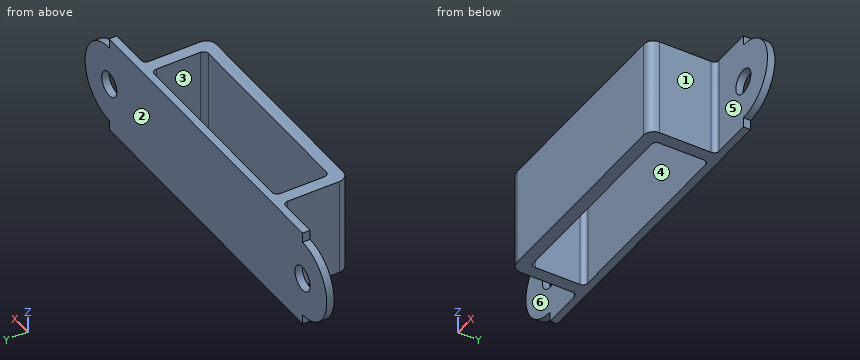
```python
from build123d import *

# Parameters (mm, degrees)
F0_W     = 46
F0_H     = 10
F1_DEPTH = 1.5
F2_DEPTH = 15
F3_W     = 41
F3_H     = 11
F4_DEPTH = 12.5
F5_D     = 5
F6_R     = 1
F7_R     = 2


with BuildPart() as f1:
    # F0 (on Front) → F1 (new body)
    with BuildSketch(Plane.XZ):
        with Locations((0, -5)):
            Rectangle(F0_W, F0_H)
        with Locations((0, 5)):
            Rectangle(F0_W, F0_H)
        Polygon((32, 10), (23, 10), (23, 0), (23, -10), (32, -10), (32, -8), (32, 8), align=None)
        with BuildLine():
            ThreePointArc((32, -8), (40, 0), (32, 8))
            Line((32, 8), (32, -8))
        make_face()
        Polygon((-23, 10), (-32, 10), (-32, 8), (-32, -8), (-32, -10), (-23, -10), (-23, 0), align=None)
        with BuildLine():
            Line((-32, -8), (-32, 8))
            ThreePointArc((-32, 8), (-40, 0), (-32, -8))
        make_face()
    extrude(amount=F1_DEPTH)

    # F0 (on Front) → F2 (join)
    with BuildSketch(Plane.XZ):
        with Locations((0, -5)):
            Rectangle(F0_W, F0_H)
        with Locations((0, 5)):
            Rectangle(F0_W, F0_H)
    extrude(amount=F2_DEPTH)

    # F3 (on Top) → F4 (cut, symmetric)
    with BuildSketch(Plane.XY):
        with Locations((0, -7)):
            Rectangle(F3_W, F3_H)
    extrude(amount=F4_DEPTH, both=True, mode=Mode.SUBTRACT)

    # F5 (through all)
    with Locations(Plane(origin=(0, 0, 0), x_dir=(1, 0, 0), z_dir=(0, 1, 0))):
        with Locations((-32, 0), (32, 0)):
            Hole(F5_D / 2)

    # F6
    f6_edges = [f1.edges().sort_by_distance(p)[0] for p in [
        (-23, -1.5, 0),
        (-20.5, -1.5, 0),
        (23, -1.5, 0),
        (20.5, -1.5, 0),
        (-20.5, -12.5, 0),
        (20.5, -12.5, 0),
    ]]
    fillet(f6_edges, radius=F6_R)

    # F7
    f7_edges = [f1.edges().sort_by_distance(p)[0] for p in [
        (-23, -15, 0),
        (23, -15, 0),
    ]]
    fillet(f7_edges, radius=F7_R)


solid = f1.part
```
Work out the finished part from the listing and answer in its coordinate system (mm). Face numbers are marked on the shaded views. A direction names the side the tool comes from. Round coordinates to 2 decimals unless told otherwise and drop trailing zeros. Write each loop counter-clockwise with the first axis right and the second up, starting at its lowest first coordinate (ties: lowest second). Pieces come first, ordered by that corner, then holes.
1) A cutting plane is placed at D-D on z = 4.5. Determine the outline of the cut face in (x, y).
2) A cutting plane is placed at B-B on z = 0. Determine the outline of the cut face in (x, y).
3) Determine the mould class of the marked faces 1, 2 and 3 for opening direction Y: pulls with the +Y half, pulls with the -Y half, needs draft (parallel to the pull), parting line crosses it, or undercut.
4) A cutting plane is placed at A-A on y = -10. Determine the outline of the cut face in (x, z), and give its area (3 significant figures).
5) Consider probe 1 along Y at (x, z) = (1, -7); probe 2 along X at (y, z) = (-7.5, -6.75); probe 3 along X at (y, z) = (-1.25, 2.25). Determine where each line is inside the solid, lowest interval first.
6) Which of the six approach directions +Z, -Z, +X, -X, +Y, -Y give full straight-line access (tool end or side, diameter ignored) to the marked faces 4, 5 and 6?
7) A cutting plane is placed at C-C on x = 18. Determine the outline of the cut face in (y, z).
8) Flat-ended cylindrical pins translate along their axes: P1, Ø3, axis at y = -6, z = -4, coming from the +X side; P2, Ø2, axis at x = -31.5, z = -7.5, coming from the -Y side; P3, Ø1.6, axis at y = -1, z = 9, coming from the +X side; P4, Ø4.5, axis at x = -32, z = 0, coming from the -Y side. Find the tip coordinate at first contact, or state that the pin passes through.
Entries:
1. outline: (-38.61, -1.5) - (-24, -1.5) arc R1 cw to (-23, -2.5) - (-23, -13) arc R2 ccw to (-21, -15) - (21, -15) arc R2 ccw to (23, -13) - (23, -2.5) arc R1 cw to (24, -1.5) - (38.61, -1.5) - (38.61, 0) - (-38.61, 0) - close; hole (-20.5, -11.5) arc R1 ccw to (-19.5, -12.5) - (19.5, -12.5) arc R1 ccw to (20.5, -11.5) - (20.5, -2.5) arc R1 ccw to (19.5, -1.5) - (-19.5, -1.5) arc R1 ccw to (-20.5, -2.5) - close
2. outline: (-40, -1.5) - (-34.5, -1.5) - (-34.5, 0) - (-40, 0) - close; (-29.5, -1.5) - (-24, -1.5) arc R1 cw to (-23, -2.5) - (-23, -13) arc R2 ccw to (-21, -15) - (21, -15) arc R2 ccw to (23, -13) - (23, -2.5) arc R1 cw to (24, -1.5) - (29.5, -1.5) - (29.5, 0) - (-29.5, 0) - close; (34.5, -1.5) - (40, -1.5) - (40, 0) - (34.5, 0) - close; hole (-20.5, -11.5) arc R1 ccw to (-19.5, -12.5) - (19.5, -12.5) arc R1 ccw to (20.5, -11.5) - (20.5, -2.5) arc R1 ccw to (19.5, -1.5) - (-19.5, -1.5) arc R1 ccw to (-20.5, -2.5) - close
3. face 1: needs draft
3. face 2: pulls with the +Y half
3. face 3: undercut
4. outline: (-23, -10) - (-20.5, -10) - (-20.5, 10) - (-23, 10) - close; (20.5, -10) - (23, -10) - (23, 10) - (20.5, 10) - close
4. area: 100 mm2
5. probe 1: y = -15 to -12.5, -1.5 to 0
5. probe 2: x = -23 to -20.5, 20.5 to 23
5. probe 3: x = -39.68 to -33.09, -30.91 to 30.91, 33.09 to 39.68
6. face 4: +Z, -Z
6. face 5: +Z, -Z, +X, -Y
6. face 6: +Z, -Z, -X, -Y
7. outline: (-15, -10) - (-12.5, -10) - (-12.5, 10) - (-15, 10) - close; (-1.5, -10) - (0, -10) - (0, 10) - (-1.5, 10) - close
8. P1: stops at x = 23
8. P2: stops at y = -1.5
8. P3: stops at x = 32
8. P4: passes through
